Geometry: final body of the model. Coordinates: model frame, mm. Face numbers are marked on the shaded views. A direction names the side the tool comes from. Coordinates: 2 decimals unless noted, no trailing zeros. Write each loop counter-clockwise with the first axis right and the second up, starting at its lowest first coordinate (ties: lowest second). Pieces come first, ordered by that corner, then holes. Notation, with made-up numbers: (39.25, -4) -> (94.25, -4) arc R19 cw to (94.25, 12) -> close; hole circle Ø6 at (58, 68). An arc over 180 degrees is marked (long way). One line per item, written item: value.
```python
from build123d import *

# Parameters (mm, degrees)
F1_DEPTH = 45


with BuildPart() as f1:
    # F0 (on Front) → F1 (new body)
    with BuildSketch(Plane.XZ):
        with BuildLine():
            Line((12.5, -90), (40, -90))
            Line((40, -90), (40, 50))
            ThreePointArc((40, 50), (28.284271, 78.284271), (0, 90))
            ThreePointArc((0, 90), (-28.284271, 78.284271), (-40, 50))
            Line((-40, 50), (-40, -90))
            Line((-40, -90), (-12.5, -90))
            Line((-12.5, -90), (-12.5, 35))
            ThreePointArc((-12.5, 35), (-11.035534, 38.535534), (-7.5, 40))
            Line((-7.5, 40), (7.5, 40))
            ThreePointArc((7.5, 40), (11.035534, 38.535534), (12.5, 35))
            Line((12.5, 35), (12.5, -90))
        make_face()
    extrude(amount=F1_DEPTH)


solid = f1.part
```
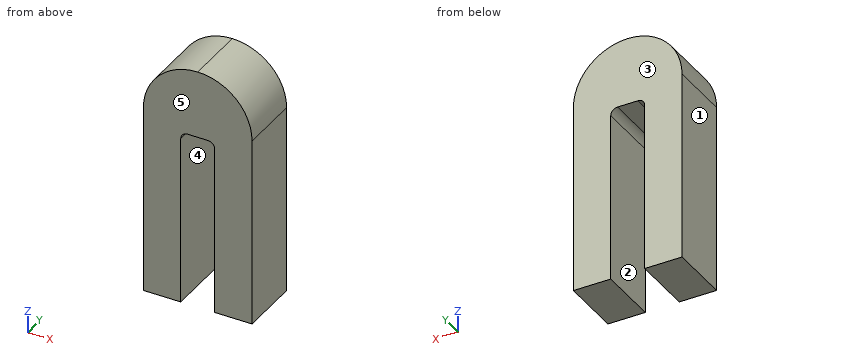
(1) Pull-direction query (X, two-part tool) for the marked faces 1, 2 and 3; classes: released by +X, released by -X, zero draft, split by the parting line, or undercut.
Responses:
face 1: released by -X
face 2: undercut
face 3: zero draft
(2) Section B-B (y = -37). Return the cut outline in (x, z).
Responses:
outline: (-40, -90) -> (-12.5, -90) -> (-12.5, 35) arc R5 cw to (-7.5, 40) -> (7.5, 40) arc R5 cw to (12.5, 35) -> (12.5, -90) -> (40, -90) -> (40, 50) arc R40 ccw to (0, 90) arc R40 ccw to (-40, 50) -> close
(3) Line query: line 1 (X direction, y = -15, z = -54.5); line 2 (X direction, y = -15.5, z = 51); line 3 (Z direction, x = 0.5, y = -23). Output: solid intervals per line, ascending. Write a range as [from, to].
Responses:
line 1: x = [-40, -12.5], [12.5, 40]
line 2: x = [-39.99, 39.99]
line 3: z = [40, 90]
(4) First-contact query: pin 1 (8 mm diameter, centred on y = -7, z = 67.5, fed in from -X); pin 2 (12 mm diameter, centred on x = -1.5, y = -33.5, fed in from -Z); pin 3 (10 mm diameter, centred on y = -7, z = 56, fed in from +X); pin 4 (12 mm diameter, centred on x = -4, y = -18, fed in from +Z). Flat tips, straight axial feed; report the tip coordinate or a pass-through.
Responses:
pin 1: stops at x = -37.65
pin 2: stops at z = 40
pin 3: stops at x = 39.99
pin 4: stops at z = 90
(5) Section A-A (z = -28). Return the cut outline in (x, y), then the cut area to 4 significant figures.
Responses:
outline: (-40, -45) -> (-12.5, -45) -> (-12.5, 0) -> (-40, 0) -> close; (12.5, -45) -> (40, -45) -> (40, 0) -> (12.5, 0) -> close
area: 2,475 mm2
(6) Section C-C (x = 26). Return the cut outline in (y, z).
Responses:
outline: (-45, -90) -> (0, -90) -> (0, 80.4) -> (-45, 80.4) -> close
(7) Section D-D (z = 78). Return the cut outline in (x, y), then the cut area to 3 significant figures.
Responses:
outline: (-28.57, -45) -> (28.57, -45) -> (28.57, 0) -> (-28.57, 0) -> close
area: 2,570 mm2
(8) Reachability of the marked faces 4 and 5 from +Z, -Z, +X, -X, +Y, -Y: full face, straight path, thin tool, end or side. Return the list, or none.
Responses:
face 4: -Z, +Y, -Y
face 5: +Z, -Z, +X, -X, -Y
